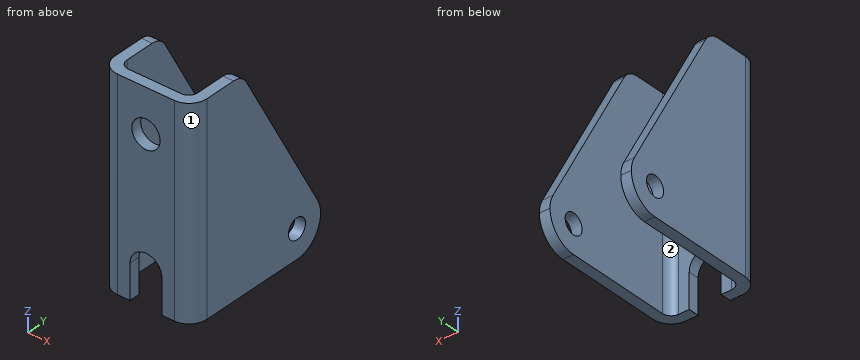
from build123d import *

# Parameters (mm, degrees)
BOSS_EXTRUDE1_DEPTH = 58.42
FILLET1_R           = 2.54
FILLET2_R           = 5.08
CUT_EXTRUDE1_START  = -26.416
CUT_EXTRUDE1_DEPTH  = 26.416
CUT_EXTRUDE2_START  = -26.416
CUT_EXTRUDE2_DEPTH  = 26.416
SKETCH2_5_R         = 2.921
CUT_EXTRUDE3_DEPTH  = 58.42
FILLET3_R           = 5.08
SKETCH4_R           = 4.064
CUT_EXTRUDE4_DEPTH  = 58.42


# Read off the part's stored shape, not the designer's step: Cut-Extrude1, Cut-Extrude2
with BuildPart() as part:
    # Sketch1 → Boss-Extrude1 (new body)
    with BuildSketch(Plane.XY):
        Polygon((-15.613299977, -11.899049236), (10.802700023, -11.899049236), (10.802700023, 32.296950764), (7.754700023, 32.296950764), (7.754700023, -8.851049236), (-12.565299977, -8.851049236), (-12.565299977, 32.296950764), (-15.613299977, 32.296950764), align=None)
    extrude(amount=-BOSS_EXTRUDE1_DEPTH)

    # Fillet1
    fillet1_edges = [part.edges().sort_by_distance(p)[0] for p in [
        (-12.565299977, -8.851049236, -29.21),
        (7.754700023, -8.851049236, -29.21),
    ]]
    fillet(fillet1_edges, radius=FILLET1_R)

    # Fillet2
    fillet2_edges = [part.edges().sort_by_distance(p)[0] for p in [
        (10.802700023, -11.899049236, -29.21),
        (-15.613299977, -11.899049236, -29.21),
    ]]
    fillet(fillet2_edges, radius=FILLET2_R)

    # Cut-Extrude1 outline → Cut-Extrude1 (cut)
    with BuildSketch(Plane(origin=(10.802700023, 0, 0), x_dir=(0, 0, -1), z_dir=(1, 0, 0)).offset(CUT_EXTRUDE1_START)):
        with BuildLine():
            Line((0, 32.296950764), (0, 5.372950764))
            Line((0, 5.372950764), (46.326645987, 31.26409951))
            ThreePointArc((46.326645987, 31.26409951), (48.229617736, 32.030995509), (50.263996941, 32.296950764))
            Line((50.263996941, 32.296950764), (0, 32.296950764))
        make_face()
    extrude(amount=CUT_EXTRUDE1_DEPTH, mode=Mode.SUBTRACT)

    # Cut-Extrude2 outline → Cut-Extrude2 (cut)
    with BuildSketch(Plane(origin=(10.802700023, 0, 0), x_dir=(0, 0, -1), z_dir=(1, 0, 0)).offset(CUT_EXTRUDE2_START)):
        with BuildLine():
            ThreePointArc((50.320003059, 32.296950764), (56.039398027, 29.916348791), (58.42, 24.196953823))
            Line((58.42, 24.196953823), (58.42, 32.296950764))
            Line((58.42, 32.296950764), (50.320003059, 32.296950764))
        make_face()
    extrude(amount=CUT_EXTRUDE2_DEPTH, mode=Mode.SUBTRACT)

    # Sketch2<5> → Cut-Extrude3 (cut)
    with BuildSketch(Plane(origin=(10.802700023, 0, 0), x_dir=(0, 0, -1), z_dir=(1, 0, 0))):
        with Locations((50.292, 24.168950764)):
            Circle(SKETCH2_5_R)
    extrude(amount=-CUT_EXTRUDE3_DEPTH, mode=Mode.SUBTRACT)

    # Fillet3
    fillet3_edges = [part.edges().sort_by_distance(p)[0] for p in [
        (-14.089299977, 5.372950764, 0),
        (9.278700023, 5.372950764, 0),
    ]]
    fillet(fillet3_edges, radius=FILLET3_R)

    # Sketch4 → Cut-Extrude4 (cut)
    with BuildSketch(Plane(origin=(0, -11.899049236, 0), x_dir=(-1, 0, 0), z_dir=(0, -1, 0))):
        with Locations(Location((2.405299977, 12.446, 0), (0, 0, 90))):
            Circle(SKETCH4_R)
        with BuildLine():
            ThreePointArc((-2.166700023, 48.514), (2.405299977, 43.942), (6.977299977, 48.514))
            Line((6.977299977, 48.514), (6.977299977, 58.42))
            Line((6.977299977, 58.42), (-2.166700023, 58.42))
            Line((-2.166700023, 58.42), (-2.166700023, 48.514))
        make_face()
    extrude(amount=-CUT_EXTRUDE4_DEPTH, mode=Mode.SUBTRACT)


solid = part.part
Source: CAD feature listing. Evaluate the final solid. Frame: model axes, mm. Face numbers are marked on the shaded views. A direction names the side the tool comes from. Round coordinates to 2 decimals unless told otherwise and drop trailing zeros. Write each loop counter-clockwise with the first axis right and the second up, starting at its lowest first coordinate (ties: lowest second). Pieces come first, ordered by that corner, then holes. Notation, with made-up numbers: M 22.25,69.25 L 80.25,69.25 A18 cw 80.25,86.25 Z; hole C 29,2.25 d3. An arc over 180 degrees is marked long. One line per item, written item: value. Start each with the question number.
Item 1: Set-up query: the marked faces 1 and 2. Return all of +Z, -Z, +X, -X, +Y, -Y with unobstructed straight access to the full face (end or side cutting, diameter ignored); none if empty.
Item 2: Ray query, L1, parallel to X at y = -4, z = -17; L2, parallel to Y at x = -4.25, z = -37; L3, parallel to Y at x = 5.5, z = -32. Return the intervals inside material, ascending. Write a range as from..to.
Item 3: Section query A-A (y = 1). Return the cut outline in (x, z), plus the area to 3 significant figures.
Item 4: Section query B-B (x = -5.5). Return the cut outline in (y, z).
Item 5: Section query C-C (z = -13). Return the cut outline in (x, y).
Item 6: Section query D-D (z = -37). Return the cut outline in (x, y).
Item 7: Pin query (flat end, axial travel): pin 1 (1.5 mm diameter, centred on y = -9.5, z = -51.5, fed in from -X); pin 2 (6.5 mm diameter, centred on x = -2.41, z = -12.45, fed in from +Y); pin 3 (4 mm diameter, centred on x = -10, z = -47, fed in from +Y); pin 4 (7.5 mm diameter, centred on x = -1, z = -43.5, fed in from +Y). Return the tip coordinate at first contact, or that it passes through.
Result set:
1. face 1: +Z, -Z, +X, -Y
1. face 2: +Z, -Z, +Y
2. L1: x = -15.61..-12.57, 7.75..10.8
2. L2: y = -11.9..-8.85
2. L3: y = -11.9..-8.83
3. outline: M -15.61,-58.42 L -12.57,-58.42 L -12.57,0 L -15.61,0 Z; M 7.75,-58.42 L 10.8,-58.42 L 10.8,0 L 7.75,0 Z
3. area: 356 mm²
4. outline: M -11.9,-45.15 L -8.85,-45.15 L -8.85,-15.08 L -11.9,-15.08 Z; M -11.9,-9.81 L -8.85,-9.81 L -8.85,0 L -11.9,0 Z
5. outline: M -15.61,-6.82 A5.08 ccw -10.53,-11.9 L -6.43,-11.9 L -6.43,-8.85 L -10.03,-8.85 A2.54 cw -12.57,-6.31 L -12.57,12.64 L -15.61,12.64 Z; M 1.62,-11.9 L 5.72,-11.9 A5.08 ccw 10.8,-6.82 L 10.8,12.64 L 7.75,12.64 L 7.75,-6.31 A2.54 cw 5.21,-8.85 L 1.62,-8.85 Z
6. outline: M -15.61,-6.82 A5.08 ccw -10.53,-11.9 L 5.72,-11.9 A5.08 ccw 10.8,-6.82 L 10.8,26.05 L 7.75,26.05 L 7.75,-6.31 A2.54 cw 5.21,-8.85 L -10.03,-8.85 A2.54 cw -12.57,-6.31 L -12.57,26.05 L -15.61,26.05 Z
7. pin 1: stops at x = -15.23
7. pin 2: passes through
7. pin 3: stops at y = -7.91
7. pin 4: stops at y = -8.85
